Input: part model. Units: mm. Frame: model coordinates. A direction names the side the tool comes from. Give positions to 0.01 mm unless a question says otherwise; leave off trailing zeros. Loops run counter-clockwise (first coordinate to the right, second up) from the corner with the lowest first, then second, coordinate; pieces in that order, holes last. Notation, with made-up numbers: (-7, 76) -> (26, 76) arc R25 ccw to (26, 104) -> close; hole circle Ø11 at (77, -4). An arc over 180 degrees is marked (long way). Answer as a JSON object with one key per item and string values.
```python
from build123d import *

# Parameters (mm, degrees)
SKETCH1_W           = 76.2
SKETCH1_H           = 139.7
BOSS_EXTRUDE1_DEPTH = 177.8
SKETCH2_W           = 68.58
SKETCH2_H           = 135.89
CUT_EXTRUDE1_DEPTH  = 173.99
SKETCH3_W           = 144.78
SKETCH3_H           = 17.78
CUT_EXTRUDE2_DEPTH  = 1.27
SKETCH5_W           = 3.81
SKETCH5_H           = 68.58
BOSS_EXTRUDE2_DEPTH = 76.2


with BuildPart() as part:
    # Sketch1 → Boss-Extrude1 (new body)
    with BuildSketch(Plane.YZ):
        with Locations((38.1, 69.85)):
            Rectangle(SKETCH1_W, SKETCH1_H)
    extrude(amount=BOSS_EXTRUDE1_DEPTH)

    # Sketch2 → Cut-Extrude1 (cut)
    with BuildSketch(Plane.YZ.offset(177.8)):
        with Locations((38.1, 71.755)):
            Rectangle(SKETCH2_W, SKETCH2_H)
    extrude(amount=-CUT_EXTRUDE1_DEPTH, mode=Mode.SUBTRACT)

    # Sketch3 → Cut-Extrude2 (cut)
    with BuildSketch(Plane.XY.offset(3.81)):
        with Locations((96.52, 38.1)):
            Rectangle(SKETCH3_W, SKETCH3_H)
    extrude(amount=-CUT_EXTRUDE2_DEPTH, mode=Mode.SUBTRACT)

    # Sketch5 → Boss-Extrude2 (add)
    with BuildSketch(Plane.XY.offset(3.81)):
        with Locations((175.895, 38.1)):
            Rectangle(SKETCH5_W, SKETCH5_H)
    extrude(amount=BOSS_EXTRUDE2_DEPTH)


solid = part.part
```
Q1. Ray query, line 1 along Y through (x, z) = (72, 67.5); line 2 along X through (y, z) = (24.5, 69); line 3 along Z through (x, y) = (88, 60). Return the intervals inside material, ascending.
Evaluation:
{"line 1": "y = 0 to 3.81, 72.39 to 76.2", "line 2": "x = 0 to 3.81, 173.99 to 177.8", "line 3": "z = 0 to 3.81"}
Q2. Draft query along Y for faces 4 (the flat face through (88, 0, 69)), 5 (the flat face through (3.81, 38, 73)), 6 (the flat face through (0, 38, 71)), 7 (the flat face through (173.99, 38, 41)). Return one class per face: +Y half, -Y half, draft (parallel to the pull), parting line (faces both ways), or undercut.
Evaluation:
{"face 4": "-Y half", "face 5": "undercut", "face 6": "draft", "face 7": "undercut"}
Q3. Section D-D, the plane z = 123.5. Return the cut outline in (x, y), then the cut area to 3 significant figures.
Evaluation:
{"outline": "(0, 0) -> (177.8, 0) -> (177.8, 3.81) -> (3.81, 3.81) -> (3.81, 72.39) -> (177.8, 72.39) -> (177.8, 76.2) -> (0, 76.2) -> close", "area": "1,620 mm2"}
Q4. Section B-B, the plane y = 8.5. Return the cut outline in (x, z), then the cut area to 3 significant figures.
Evaluation:
{"outline": "(0, 0) -> (177.8, 0) -> (177.8, 80.01) -> (173.99, 80.01) -> (173.99, 3.81) -> (3.81, 3.81) -> (3.81, 139.7) -> (0, 139.7) -> close", "area": "1,490 mm2"}
Q5. Section A-A, the plane z = 39. Return the cut outline in (x, y).
Evaluation:
{"outline": "(0, 0) -> (177.8, 0) -> (177.8, 76.2) -> (0, 76.2) -> close; hole (3.81, 3.81) -> (173.99, 3.81) -> (173.99, 72.39) -> (3.81, 72.39) -> close"}
Q6. Pin query (flat end, axial travel): pin 1 (4 mm diameter, centred on x = 89, y = 32, fed in from -Z); pin 2 (19.5 mm diameter, centred on x = 120.5, y = 40.5, fed in from +Z); pin 3 (3 mm diameter, centred on x = 175.5, y = 21.5, fed in from +Z); pin 4 (10 mm diameter, centred on x = 118.5, y = 39, fed in from +Z). Return the tip coordinate at first contact, or that it passes through.
Evaluation:
{"pin 1": "stops at z = 0", "pin 2": "stops at z = 3.81", "pin 3": "stops at z = 80.01", "pin 4": "stops at z = 2.54"}
Q7. Section C-C, the plane x = 165. Return the cut outline in (y, z), then the cut area to 3 significant figures.
Evaluation:
{"outline": "(0, 0) -> (76.2, 0) -> (76.2, 139.7) -> (72.39, 139.7) -> (72.39, 3.81) -> (46.99, 3.81) -> (46.99, 2.54) -> (29.21, 2.54) -> (29.21, 3.81) -> (3.81, 3.81) -> (3.81, 139.7) -> (0, 139.7) -> close", "area": "1,300 mm2"}
Q8. Access query for faces 1 (the flat face through (88, 76.2, 69)), 2 (the flat face through (90, 22, 3.81)), 3 (the flat face through (176, 39, 80.01)). Directions: +Z, -Z, +X, -X, +Y, -Y. A direction counts if a zero-diameter tool reaches every point of the face in a straight line with its end or side. Return the directions, or none.
Evaluation:
{"face 1": "+Z, -Z, +X, -X, +Y", "face 2": "+Z", "face 3": "+Z, +X"}
